from build123d import *

# Parameters (mm, degrees)
BOSS_EXTRUDE1_DEPTH = 10
CUT_EXTRUDE3_DEPTH  = 28.676705006
CUT_EXTRUDE6_START  = -13
CUT_EXTRUDE6_DEPTH  = 2
CUT_EXTRUDE14_START = -3
CUT_EXTRUDE14_DEPTH = 2
CUT_EXTRUDE7_START  = 10
SKETCH8_R           = 2.75
CUT_EXTRUDE7_DEPTH  = 2
CUT_EXTRUDE8_START  = -16
SKETCH10_R          = 2.25
CUT_EXTRUDE8_DEPTH  = 3
CUT_EXTRUDE9_DEPTH  = 5
SKETCH18_R          = 0.75
CUT_EXTRUDE12_DEPTH = 28.676705006
CUT_EXTRUDE13_START = 5
SKETCH19_W          = 4
SKETCH19_H          = 4
CUT_EXTRUDE13_DEPTH = 1
CUT_EXTRUDE15_START = -1
SKETCH5_R           = 1.75
CUT_EXTRUDE15_DEPTH = 2
CUT_EXTRUDE16_START = -1
CUT_EXTRUDE16_DEPTH = 2
FILLET2_R           = 0.5
FILLET3_R           = 1
POT_INSERT_DEPTH    = 2.5
POT_START           = 4
SKETCH6_R           = 2.75
POT_HOLE_DEPTH      = 1.5
SCREW_START         = 11
SKETCH14_R          = 0.8
SCREW_HOLES_DEPTH   = 9
SCREW_START_2       = 10
SKETCH15_R          = 1.25
SCREW_HEADS_DEPTH   = 2
CUT_EXTRUDE11_START = 10
SKETCH13_W          = 21
SKETCH13_H          = 15
CUT_EXTRUDE11_DEPTH = 5


with BuildPart() as part:
    # Sketch1 → Boss-Extrude1 (new body)
    with BuildSketch(Plane(origin=(0, 0, 0), x_dir=(1, 0, 0), z_dir=(0, 1, 0))):
        with BuildLine():
            Line((21, 15), (21, 8))
            Line((21, 8), (21, 1))
            Line((21, 1), (12, 1))
            Line((12, 1), (2.253205655, 1))
            ThreePointArc((2.253205655, 1), (0, 8), (2.253205655, 15))
            Line((2.253205655, 15), (12, 15))
            Line((12, 15), (21, 15))
        make_face()
    extrude(amount=BOSS_EXTRUDE1_DEPTH)

    # Sketch4 → Cut-Extrude3 (cut, through all)
    with BuildSketch(Plane.XY):
        with BuildLine():
            Line((21, 14), (12, 14))
            ThreePointArc((12, 14), (18.363961031, 11.363961031), (21, 5))
            Line((21, 5), (21, 14))
        make_face()
        with BuildLine():
            Line((21, -4), (21, 5))
            ThreePointArc((21, 5), (18.363961031, -1.363961031), (12, -4))
            Line((12, -4), (21, -4))
        make_face()
    extrude(amount=-CUT_EXTRUDE3_DEPTH, mode=Mode.SUBTRACT)

    # Sketch7 → Cut-Extrude6 (cut)
    with BuildSketch(Plane.XY.offset(CUT_EXTRUDE6_START)):
        Polygon((21, 5.5), (21, 11), (10, 11), (10, 7.5), (0, 7.5), (0, 3.5), (21, 3.5), align=None)
    extrude(amount=CUT_EXTRUDE6_DEPTH, mode=Mode.SUBTRACT)

    # Sketch21 → Cut-Extrude14 (cut)
    with BuildSketch(Plane.XY.offset(CUT_EXTRUDE14_START)):
        Polygon((21, 5.5), (21, 11), (10, 11), (10, 7.5), (0, 7.5), (0, 3.5), (21, 3.5), align=None)
    extrude(amount=-CUT_EXTRUDE14_DEPTH, mode=Mode.SUBTRACT)

    # Sketch8 → Cut-Extrude7 (cut)
    with BuildSketch(Plane(origin=(0, 0, 0), x_dir=(1, 0, 0), z_dir=(0, 1, 0)).offset(CUT_EXTRUDE7_START)):
        with Locations(Location((12, 8, 0), (0, 0, 270))):
            Circle(SKETCH8_R)
    extrude(amount=-CUT_EXTRUDE7_DEPTH, mode=Mode.SUBTRACT)

    # Sketch10 → Cut-Extrude8 (cut)
    with BuildSketch(Plane.XY.offset(CUT_EXTRUDE8_START)):
        with Locations(Location((12, 5, 0), (0, 0, 221.810314896))):
            Circle(SKETCH10_R)
    extrude(amount=CUT_EXTRUDE8_DEPTH, mode=Mode.SUBTRACT)

    # Sketch11 → Cut-Extrude9 (cut)
    with BuildSketch(Plane(origin=(0, 0, 0), x_dir=(0, 0, -1), z_dir=(1, 0, 0))):
        Polygon((8, 2), (13, 2), (13, 8), (3, 8), (3, 2), align=None)
    extrude(amount=CUT_EXTRUDE9_DEPTH, mode=Mode.SUBTRACT)

    # Sketch18 → Cut-Extrude12 (cut, through all)
    with BuildSketch(Plane.XY):
        with Locations((12, 5)):
            Circle(SKETCH18_R)
    extrude(amount=-CUT_EXTRUDE12_DEPTH, mode=Mode.SUBTRACT)

    # Sketch19 → Cut-Extrude13 (cut, symmetric)
    with BuildSketch(Plane(origin=(0, 0, 0), x_dir=(1, 0, 0), z_dir=(0, 1, 0)).offset(CUT_EXTRUDE13_START)):
        with Locations((12, 8)):
            Rectangle(SKETCH19_W, SKETCH19_H)
    extrude(amount=CUT_EXTRUDE13_DEPTH, both=True, mode=Mode.SUBTRACT)

    # Sketch5 → Cut-Extrude15 (cut)
    with BuildSketch(Plane.XY.offset(CUT_EXTRUDE15_START)):
        with Locations((12, 5)):
            Circle(SKETCH5_R)
    extrude(amount=-CUT_EXTRUDE15_DEPTH, mode=Mode.SUBTRACT)

    # Sketch26 → Cut-Extrude16 (cut)
    with BuildSketch(Plane.XY.offset(CUT_EXTRUDE16_START)):
        with BuildLine():
            Line((16.483314774, 10), (19.483314774, 10))
            ThreePointArc((19.483314774, 10), (20.800790614, 6.883105034), (20.874119675, 3.5))
            Line((20.874119675, 3.5), (17.874119675, 3.5))
            ThreePointArc((17.874119675, 3.5), (17.800790614, 6.883105034), (16.483314774, 10))
        make_face()
    extrude(amount=-CUT_EXTRUDE16_DEPTH, mode=Mode.SUBTRACT)

    # Fillet2
    fillet2_edges = [part.edges().sort_by_distance(p)[0] for p in [
        (12, 8, -10.75),
    ]]
    fillet(fillet2_edges, radius=FILLET2_R)

    # Fillet3
    # the kernel refuses this fillet: 1 mm, written as the material it takes off along each edge
    with BuildSketch(Plane(origin=(12, 5, -13), x_dir=(0.6472427025312245, 0.7622839917118008, 0), z_dir=(-0.7622839917118008, 0.6472427025312245, 0))) as fillet3_piece_1_section:
        with BuildLine():
            CenterArc((9 - FILLET3_R, FILLET3_R), FILLET3_R, 270, 90)
            Line((9 - FILLET3_R, 0), (9, 0))
            Line((9, 0), (9, FILLET3_R))
        make_face()
    fillet3_piece_1 = revolve(axis=Axis((12, 5, -13), (0, 0, -1)), revolution_arc=75.177010416, mode=Mode.PRIVATE)
    fillet3_piece_1 = split(fillet3_piece_1, bisect_by=Plane(origin=(20.22008164, 3.5, -13.28352735), z_dir=(0, 1, 0)), keep=Keep.TOP, mode=Mode.PRIVATE)
    add(fillet3_piece_1, mode=Mode.SUBTRACT)
    with BuildSketch(Plane(origin=(12, 5, -11), x_dir=(0.9025022770828605, -0.43068508200337235, 0), z_dir=(-0.43068508200337235, -0.9025022770828605, 0))) as fillet3_piece_2_section:
        with BuildLine():
            CenterArc((9 - FILLET3_R, FILLET3_R), FILLET3_R, 270, 90)
            Line((9 - FILLET3_R, 0), (9, 0))
            Line((9, 0), (9, FILLET3_R))
        make_face()
    fillet3_piece_2 = revolve(axis=Axis((12, 5, -11), (0, 0, 1)), revolution_arc=75.177010416, mode=Mode.PRIVATE)
    fillet3_piece_2 = split(fillet3_piece_2, bisect_by=Plane(origin=(20.220081643, 3.5, -10.716472653), z_dir=(0, 1, 0)), keep=Keep.TOP, mode=Mode.PRIVATE)
    add(fillet3_piece_2, mode=Mode.SUBTRACT)
    with BuildSketch(Plane(origin=(21.983314774, 10, -11), x_dir=(0, 0, 1), z_dir=(-1, 0, 0))) as fillet3_piece_3:
        with BuildLine():
            CenterArc((FILLET3_R, -FILLET3_R), FILLET3_R, 90, 90)
            Line((0, -FILLET3_R), (0, 0))
            Line((0, 0), (FILLET3_R, 0))
        make_face()
    extrude(amount=11.983314774, mode=Mode.SUBTRACT)
    with BuildSketch(Plane(origin=(21.983314774, 10, -13), x_dir=(0, 0, -1), z_dir=(-1, 0, 0))) as fillet3_piece_4:
        with BuildLine():
            CenterArc((FILLET3_R, FILLET3_R), FILLET3_R, 180, 90)
            Line((0, FILLET3_R), (0, 0))
            Line((0, 0), (FILLET3_R, 0))
        make_face()
    extrude(amount=11.983314774, mode=Mode.SUBTRACT)

    # Sketch3 → Pot Insert (cut)
    with BuildSketch(Plane(origin=(28.28760271, 0, 0), x_dir=(1, 0, 0), z_dir=(0, 1, 0))):
        Polygon((-25.28760271, 12.5), (-20.53760271, 12.5), (-20.53760271, 13.5), (-16.28760271, 13.5), (-12.291072924, 13.5), (-12.291072924, 12.500096395), (-10.791072924, 9.500096395), (-9.28760271, 9.500096395), (-9.28760271, 8), (-9.28760271, 6.5), (-10.78760271, 6.5), (-12.28760271, 3.5), (-12.28760271, 2.5), (-16.28760271, 2.5), (-20.53760271, 2.5), (-20.53760271, 3.5), (-25.28760271, 3.5), (-25.28760271, 8), align=None)
    extrude(amount=POT_INSERT_DEPTH, mode=Mode.SUBTRACT)

    # Sketch6 → Pot Hole (cut)
    with BuildSketch(Plane(origin=(0, 0, 0), x_dir=(1, 0, 0), z_dir=(0, 1, 0)).offset(POT_START)):
        with Locations(Location((12, 8, 0), (0, 0, 270))):
            Circle(SKETCH6_R)
    extrude(amount=-POT_HOLE_DEPTH, mode=Mode.SUBTRACT)

    # Sketch14 → Screw Holes (cut)
    with BuildSketch(Plane(origin=(0, 0, 0), x_dir=(1, 0, 0), z_dir=(0, 1, 0)).offset(SCREW_START)):
        with Locations(Location((7, 8, 0), (0, 0, 270))):
            Circle(SKETCH14_R)
        with Locations(Location((17, 8, 0), (0, 0, 270))):
            Circle(SKETCH14_R)
    extrude(amount=-SCREW_HOLES_DEPTH, mode=Mode.SUBTRACT)

    # Sketch15 → Screw Heads (cut)
    with BuildSketch(Plane(origin=(0, 0, 0), x_dir=(1, 0, 0), z_dir=(0, 1, 0)).offset(SCREW_START_2)):
        with Locations(Location((7, 8, 0), (0, 0, 270))):
            Circle(SKETCH15_R)
        with Locations(Location((17, 8, 0), (0, 0, 270))):
            Circle(SKETCH15_R)
    extrude(amount=-SCREW_HEADS_DEPTH, mode=Mode.SUBTRACT)

    # Sketch13 → Cut-Extrude11 (cut)
    with BuildSketch(Plane(origin=(0, 0, 0), x_dir=(1, 0, 0), z_dir=(0, 1, 0)).offset(CUT_EXTRUDE11_START)):
        with Locations((10.5, 7.5)):
            Rectangle(SKETCH13_W, SKETCH13_H)
    extrude(amount=-CUT_EXTRUDE11_DEPTH, mode=Mode.SUBTRACT)


solid = part.part
Design review of the part built by this model. Coordinates are the model's own, in mm. A direction names the side the tool comes from. Give positions to 0.01 mm unless a question says otherwise; leave off trailing zeros. Write each loop counter-clockwise with the first axis right and the second up, starting at its lowest first coordinate (ties: lowest second). Pieces come first, ordered by that corner, then holes. Notation, with made-up numbers: M -28.75,81 L 1.25,81 A17 ccw 1.25,114 Z; hole C 25.25,25.25 d2. An arc over 180 degrees is marked long. Return JSON: item names as keys, results as strings. Group by question number.
Item 1: Take a section at C-C (y = 1.5). Give the boundary of the cut face in (x, z).
Item 2: Tool access review of faces 1 (the flat face through (5, 4, -3)), 2 (the flat face through (12, 1, -13.5)), 3 (the cylindrical face through (16.51, 3.77, -8.63)), 4 (the flat face through (13, 4, -5)): name each direction out of +Z, -Z, +X, -X, +Y, -Y from which nothing blocks a thin tool from reaching the whole face with its end or side.
Item 3: The part is to be moulded in two halves that separate along X. For faces 5 (the flat face through (17, 4, -13)), 6 (the cylindrical face through (20.436, 1.865, -7.902)), 7 (the cylindrical face through (11.96, 3.25, -1.99)), say which applies: pulls with the +X half, pulls with the -X half, needs draft (parallel to the pull), parting line crosses it, or undercut.
Item 4: Clearance check with flat-ended pins moving along their axes: pin 1 Ø2 at (y, z) = (3, -3.5) entering from +X; pin 2 Ø0.6 at (x, z) = (9.5, -7) entering from -Y; pin 3 Ø0.5 at (y, z) = (1, -3) entering from -X; pin 4 Ø4 at (x, z) = (18, -7) entering from -Y. State where each tip first meets the part, or that it passes through.
Item 5: Wall thickness on line 1 along Z through (x, y) = (8, 3.7); line 2 along Z through (x, y) = (12, 2.9); line 3 along Z through (x, y) = (3.5, 2.1): over which ranges is each line inside the solid? List them lowest first.
Item 6: Take a section at D-D (z = -4). Give the boundary of the cut face in (x, y).
Item 7: Take a section at B-B (z = -8). Give the boundary of the cut face in (x, y).
Item 8: Take a section at A-A (x = 4.5). Give the boundary of the cut face in (y, z).
Return value:
{
 "1": {"outline": "M 2.25,-15 L 20.29,-15 L 20.29,-1 L 2.25,-1 A12 ccw Z; hole M 3,-12.5 L 7.75,-12.5 L 7.75,-13.5 L 16,-13.5 L 16,-12.5 L 17.5,-9.5 L 19,-9.5 L 19,-6.5 L 17.5,-6.5 L 16,-3.5 L 16,-2.5 L 7.75,-2.5 L 7.75,-3.5 L 3,-3.5 Z"},
 "2": {"face 1": "-X, +Y", "face 2": "-Y", "face 3": "+Y, -Y", "face 4": "+X, -X, +Y"},
 "3": {"face 5": "needs draft", "face 6": "pulls with the +X half", "face 7": "undercut"},
 "4": {"pin 1": "stops at x = 20.87", "pin 2": "stops at y = 2.5", "pin 3": "stops at x = 0.98", "pin 4": "stops at y = 0"},
 "5": {"line 1": "z = -15 to -13, -11 to -5, -3 to -1", "line 2": "z = -13 to -10.75, -5.25 to -1", "line 3": "z = -15 to -13, -3 to -1"},
 "6": {"outline": "M 0.69,0 L 3,0 L 3,2 L 0.69,2 Z; M 5,2.5 L 16.25,2.5 L 16.25,0 L 19.48,0 A9 ccw 20.87,3.5 L 5,3.5 Z"},
 "7": {"outline": "M 0,0 L 3,0 L 3,2 L 0,2 Z; M 5,2.5 L 6.2,2.5 L 6.2,5 L 5,5 Z; M 7.8,2.5 L 9.25,2.5 L 9.25,4 L 10,4 L 10,5 L 7.8,5 Z; M 14,4 L 14.75,4 L 14.75,2.5 L 16.2,2.5 L 16.2,5 L 14,5 Z; M 17.8,2.5 L 19,2.5 L 19,0 L 19.48,0 A9 ccw 21,5 L 17.8,5 Z"},
 "8": {"outline": "M 0,-15 L 5,-15 L 5,-13 L 2,-13 L 2,-12.5 L 0,-12.5 Z; M 0,-3.5 L 2,-3.5 L 2,-3 L 5,-3 L 5,-1 L 0,-1 Z"}
}
